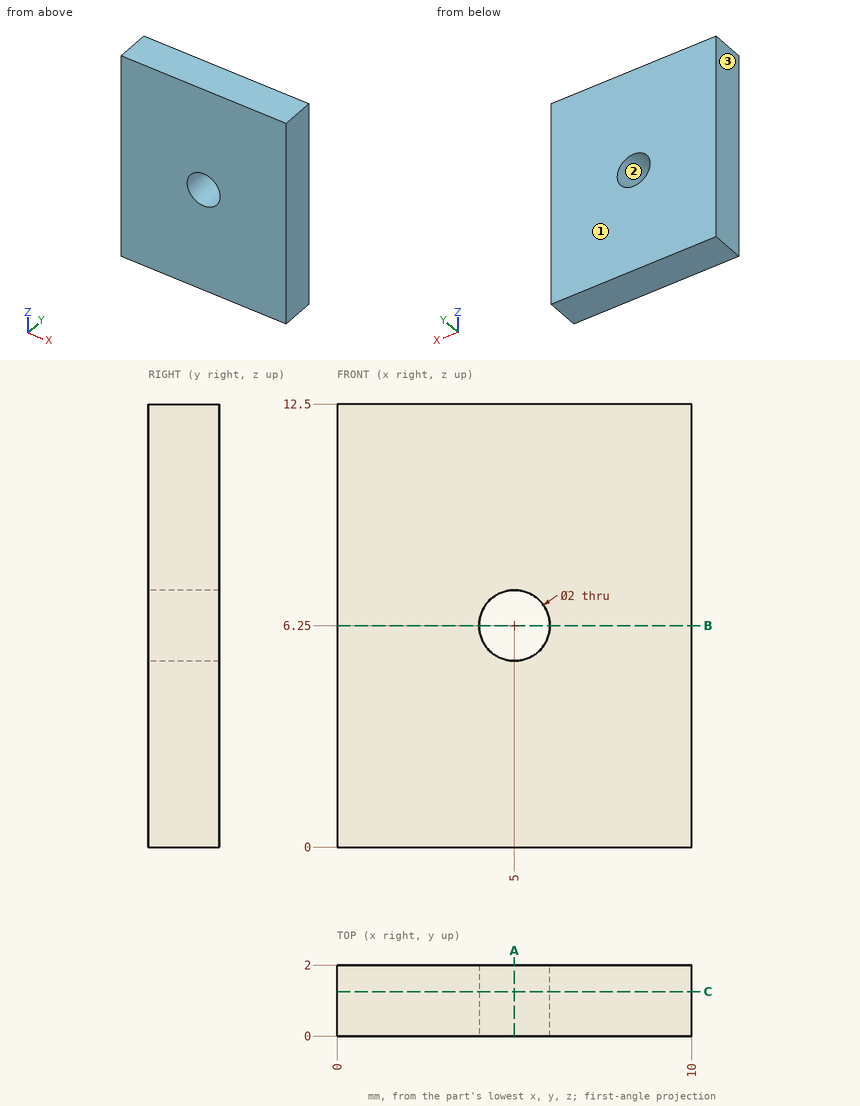
Could you check a few things on this drawing? It's one solid part, dimensions in mm from its lowest x, y, z. Round coordinates to 2 decimals unless told otherwise and drop trailing zeros. Order: outer loops, then holes, each group sorted by start corner. A loop starts at its lowest first (then second) coordinate and runs counter-clockwise, first axis right, second up. Notation, with made-up numbers: M -8,50 L 8,50 A31 cw 8,81 Z; hole C 6.5,-21 d8. An arc over 180 degrees is marked long. Return JSON: item names as keys, results as strings. Group by question number.
1. If we mould it in two halves opening along X, with no side actions, what happens to the marked faces 1, 2 and 3? For each: pulls with the +X half, pulls with the -X half, needs draft (parallel to the pull), parting line crosses it, or undercut.
2. I'm going to push a flat-ended pin straight in: pin 1 Ø1.2 at (x, z) = (5, 6.25) entering from -Y. Where does the tip first touch, or does it pass through?
3. If we section it at C-C on y = 1.25: List the corners of the cut face in (x, z) for me.
4. If we section it at B-B on z = 6.25: List the corners of the cut face in (x, y) for me.
5. Please list where these lines run through material, in increasing order: probe 1 along Z at (x, y) = (5, 1.25); probe 2 along X at (y, z) = (1.45, 6.25); probe 3 along Z at (x, y) = (4.5, 1.35).
6. If we section it at A-A on x = 5: List the corners of the cut face in (y, z) for me.
Reply:
{
 "1": {"face 1": "needs draft", "face 2": "undercut", "face 3": "pulls with the -X half"},
 "2": {"pin 1": "through"},
 "3": {"outline": "M 0,0 L 10,0 L 10,12.5 L 0,12.5 Z; hole C 5,6.25 d2"},
 "4": {"outline": "M 0,0 L 4,0 L 4,2 L 0,2 Z; M 6,0 L 10,0 L 10,2 L 6,2 Z"},
 "5": {"probe 1": "0 to 5.25, 7.25 to 12.5", "probe 2": "0 to 4, 6 to 10", "probe 3": "0 to 5.38, 7.12 to 12.5"},
 "6": {"outline": "M 0,0 L 2,0 L 2,5.25 L 0,5.25 Z; M 0,7.25 L 2,7.25 L 2,12.5 L 0,12.5 Z"}
}
